Read the model definition and answer for the solid it produces. Units are mm, in the model's axes. Face numbers are marked on the shaded views. A direction names the side the tool comes from. Give positions to 0.01 mm unless a question says otherwise; leave off trailing zeros. Loops run counter-clockwise (first coordinate to the right, second up) from the corner with the lowest first, then second, coordinate; pieces in that order, holes last.
(1) Which of the six approach directions +Z, -Z, +X, -X, +Y, -Y give full straight-line access (tool end or side, diameter ignored) to the marked faces 1, 2 and 3?
(2) Find section A-A, the plane z = 4. Write down the section's boundary in (x, y).
(3) Straight lines are drawn through the part: probe 1 along Y at (x, z) = (0, 13.5); probe 2 along Y at (x, z) = (-1, 11.25); probe 3 along X at (y, z) = (-6, 5). For each, find the intervals that lie inside material, in ascending order.
(4) Determine the mould class of the marked faces 4, 5 and 6 for opening direction Y: pulls with the +Y half, pulls with the -Y half, needs draft (parallel to the pull), parting line crosses it, or undercut.
(5) Find section C-C, the plane y = -6. Write down the section's boundary in (x, z).
(6) Each of these flat-tipped pins is pushed along its axis until it touches: P1, Ø12, axis at x = -15, y = -14, coming from the +Z side; P2, Ø10, axis at y = 11, z = 5, coming from the -X side; P3, Ø3, axis at y = -13.5, z = 10, coming from the +X side. Where does it stop, or does it pass through?
(7) Find section D-D, the plane z = 13.75. Write down the section's boundary in (x, y).
(8) Find section B-B, the plane y = 0. Write down the section's boundary in (x, z), then the cut area to 3 significant figures.
```python
from build123d import *

# Parameters (mm, degrees)
IZIM1_R                     = 8.5
Y_KSEKLIK_EKSTR_ZYON1_DEPTH = 27.5
IZIM2_R                     = 8
Y_KSEKLIK_EKSTR_ZYON3_DEPTH = 22.5


with BuildPart() as part:
    # Çizim1 → Yükseklik-Ekstrüzyon1 (new body)
    with BuildSketch(Plane.XY):
        Polygon((0, 20.784609691), (-18, 10.392304845), (-18, -10.392304845), (0, -20.784609691), (18, -10.392304845), (18, 10.392304845), align=None)
        Circle(IZIM1_R, mode=Mode.SUBTRACT)
    extrude(amount=Y_KSEKLIK_EKSTR_ZYON1_DEPTH)

    # Çizim2 → Yükseklik-Ekstrüzyon3 (add)
    with BuildSketch(Plane(origin=(18, 0, 0), x_dir=(0, 0, -1), z_dir=(1, 0, 0))):
        with Locations(Location((-13.75, 0, 0), (0, 0, 270))):
            Circle(IZIM2_R)
    y_kseklik_ekstr_zyon3 = extrude(amount=Y_KSEKLIK_EKSTR_ZYON3_DEPTH)

    # Aynalama1: Yükseklik-Ekstrüzyon3 across plane
    add(y_kseklik_ekstr_zyon3.mirror(Plane(origin=(0, 0, 0), x_dir=(0, 0, 1), z_dir=(1, 0, 0))))


solid = part.part
```
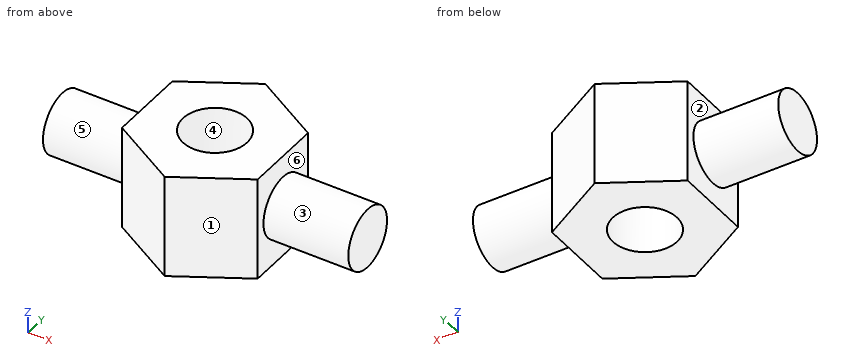
Entries:
1. face 1: +Z, -Z, +X, -Y
1. face 2: -X
1. face 3: +X
2. outline: (-18, -10.39) - (0, -20.78) - (18, -10.39) - (18, 10.39) - (0, 20.78) - (-18, 10.39) - close; hole circle Ø17 at (0, 0)
3. probe 1: y = -20.78 to -8.5, 8.5 to 20.78
3. probe 2: y = -20.21 to -8.44, 8.44 to 20.21
3. probe 3: x = -18 to -6.02, 6.02 to 18
4. face 4: undercut
4. face 5: parting line crosses it
4. face 6: needs draft
5. outline: (-40.5, 8.46) - (-18, 8.46) - (-18, 0) - (-6.02, 0) - (-6.02, 27.5) - (-18, 27.5) - (-18, 19.04) - (-40.5, 19.04) - close; (6.02, 0) - (18, 0) - (18, 8.46) - (40.5, 8.46) - (40.5, 19.04) - (18, 19.04) - (18, 27.5) - (6.02, 27.5) - close
6. P1: stops at z = 27.5
6. P2: stops at x = -18
6. P3: stops at x = 15.22
7. outline: (-40.5, -8) - (-18, -8) - (-18, -10.39) - (0, -20.78) - (18, -10.39) - (18, -8) - (40.5, -8) - (40.5, 8) - (18, 8) - (18, 10.39) - (0, 20.78) - (-18, 10.39) - (-18, 8) - (-40.5, 8) - close; hole circle Ø17 at (0, 0)
8. outline: (-40.5, 5.75) - (-18, 5.75) - (-18, 0) - (-8.5, 0) - (-8.5, 27.5) - (-18, 27.5) - (-18, 21.75) - (-40.5, 21.75) - close; (8.5, 0) - (18, 0) - (18, 5.75) - (40.5, 5.75) - (40.5, 21.75) - (18, 21.75) - (18, 27.5) - (8.5, 27.5) - close
8. area: 1,240 mm2
